Work out the finished part from the listing and answer in its coordinate system (mm). Coordinates: 2 decimals unless noted, no trailing zeros. Order: outer loops, then holes, each group sorted by start corner. A loop starts at its lowest first (then second) coordinate and runs counter-clockwise, first axis right, second up.
```python
from build123d import *

# Parameters (mm, degrees)
EXTRUDE_1_DEPTH = 1


with BuildPart() as part:
    # 草图1 → 凸台-拉伸1 (new body)
    with BuildSketch(Plane.XY):
        with BuildLine():
            Line((-4, -15), (6, -15))
            ThreePointArc((6, -15), (13.071067812, -12.071067812), (16, -5))
            Line((16, -5), (16, 70))
            Line((16, 70), (29.076696831, 92.649503306))
            Line((29.076696831, 92.649503306), (29.076696831, 147.803847577))
            Line((29.076696831, 147.803847577), (-4.776615382, 147.803847577))
            Line((-4.776615382, 147.803847577), (-14, 138.58046296))
            Line((-14, 138.58046296), (-14, -5))
            ThreePointArc((-14, -5), (-11.071067812, -12.071067812), (-4, -15))
        make_face()
        with BuildLine():
            ThreePointArc((-6.682159082, 114.682159082), (0, 98.55), (6.682159082, 114.682159082))
            Line((6.682159082, 114.682159082), (3.341079541, 118.023238623))
            ThreePointArc((3.341079541, 118.023238623), (0, 119.407159082), (-3.341079541, 118.023238623))
            Line((-3.341079541, 118.023238623), (-6.682159082, 114.682159082))
        make_face(mode=Mode.SUBTRACT)
        with BuildLine():
            ThreePointArc((-6.682159082, 141.682159082), (0, 125.55), (6.682159082, 141.682159082))
            Line((6.682159082, 141.682159082), (3.341079541, 145.023238623))
            ThreePointArc((3.341079541, 145.023238623), (0, 146.407159082), (-3.341079541, 145.023238623))
            Line((-3.341079541, 145.023238623), (-6.682159082, 141.682159082))
        make_face(mode=Mode.SUBTRACT)
        with BuildLine():
            ThreePointArc((-6.682159082, 87.682159082), (0, 71.55), (6.682159082, 87.682159082))
            Line((6.682159082, 87.682159082), (3.341079541, 91.023238623))
            ThreePointArc((3.341079541, 91.023238623), (0, 92.407159082), (-3.341079541, 91.023238623))
            Line((-3.341079541, 91.023238623), (-6.682159082, 87.682159082))
        make_face(mode=Mode.SUBTRACT)
        with BuildLine():
            ThreePointArc((3.341079541, 64.023238623), (0, 65.407159082), (-3.341079541, 64.023238623))
            Line((-3.341079541, 64.023238623), (-6.682159082, 60.682159082))
            ThreePointArc((-6.682159082, 60.682159082), (0, 44.55), (6.682159082, 60.682159082))
            Line((6.682159082, 60.682159082), (3.341079541, 64.023238623))
        make_face(mode=Mode.SUBTRACT)
        with BuildLine():
            ThreePointArc((-6.682159082, 33.682159082), (0, 17.55), (6.682159082, 33.682159082))
            Line((6.682159082, 33.682159082), (3.341079541, 37.023238623))
            ThreePointArc((3.341079541, 37.023238623), (0, 38.407159082), (-3.341079541, 37.023238623))
            Line((-3.341079541, 37.023238623), (-6.682159082, 33.682159082))
        make_face(mode=Mode.SUBTRACT)
        with BuildLine():
            ThreePointArc((3.341079541, 10.023238623), (0, 11.407159082), (-3.341079541, 10.023238623))
            Line((-3.341079541, 10.023238623), (-6.682159082, 6.682159082))
            ThreePointArc((-6.682159082, 6.682159082), (0, -9.45), (6.682159082, 6.682159082))
            Line((6.682159082, 6.682159082), (3.341079541, 10.023238623))
        make_face(mode=Mode.SUBTRACT)
        Polygon((24.076696831, 105.403847577), (21.825030781, 101.503847577), (26.32836288, 101.503847577), align=None, mode=Mode.SUBTRACT)
        Polygon((26.32836288, 131.503847577), (24.076696831, 135.403847577), (21.825030781, 131.503847577), align=None, mode=Mode.SUBTRACT)
    extrude(amount=EXTRUDE_1_DEPTH)


solid = part.part
```
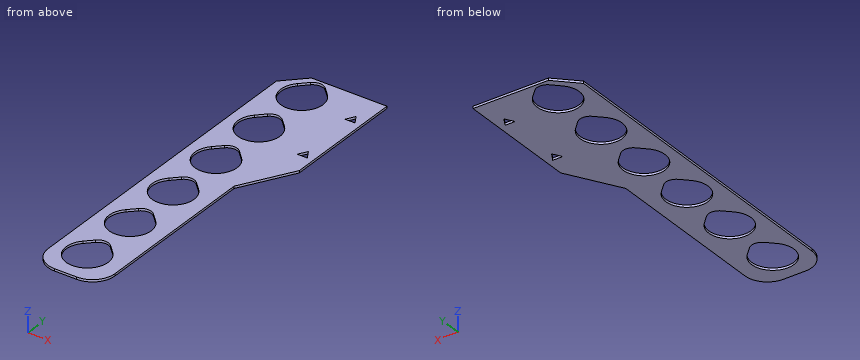
1. The part is cut by section B-B (y = 0). Determine the outline of the cut face in (x, z), plus the area to 3 significant figures.
2. The part is cut by section A-A (x = 0). Determine the outline of the cut face in (y, z), plus the area to 3 significant figures.
3. Consider probe 1 along X at (y, z) = (108, 0.75); probe 2 along X at (y, z) = (0, 0.3); probe 3 along X at (y, z) = (135, 0.75). Determine where each line is inside the solid, lowest interval first.
4. The part is cut by section C-C (y = 50). Determine the outline of the cut face in (x, z).
5. The part is cut by section D-D (x = 18.5). Determine the outline of the cut face in (y, z), plus the area to 3 significant figures.
Worked out:
1. outline: (-14, 0) - (-9.45, 0) - (-9.45, 1) - (-14, 1) - close; (9.45, 0) - (16, 0) - (16, 1) - (9.45, 1) - close
1. area: 11.1 mm2
2. outline: (-15, 0) - (-9.45, 0) - (-9.45, 1) - (-15, 1) - close; (11.41, 0) - (17.55, 0) - (17.55, 1) - (11.41, 1) - close; (38.41, 0) - (44.55, 0) - (44.55, 1) - (38.41, 1) - close; (65.41, 0) - (71.55, 0) - (71.55, 1) - (65.41, 1) - close; (92.41, 0) - (98.55, 0) - (98.55, 1) - (92.41, 1) - close; (119.41, 0) - (125.55, 0) - (125.55, 1) - (119.41, 1) - close; (146.41, 0) - (147.8, 0) - (147.8, 1) - (146.41, 1) - close
2. area: 37.7 mm2
3. probe 1: x = -14 to -9.45, 9.45 to 29.08
3. probe 2: x = -14 to -9.45, 9.45 to 16
3. probe 3: x = -14 to -9.45, 9.45 to 23.84, 24.31 to 29.08
4. outline: (-14, 0) - (-8.56, 0) - (-8.56, 1) - (-14, 1) - close; (8.56, 0) - (16, 0) - (16, 1) - (8.56, 1) - close
5. outline: (74.33, 0) - (147.8, 0) - (147.8, 1) - (74.33, 1) - close
5. area: 73.5 mm2
